Job drawing, mm, ordinate dimensions from the low corner. One solid piece. Round coordinates to 2 decimals unless told otherwise and drop trailing zeros. Write each loop counter-clockwise with the first axis right and the second up, starting at its lowest first coordinate (ties: lowest second). Pieces come first, ordered by that corner, then holes. Notation, with made-up numbers: M 4,30 L 60,30 A22 ccw 60,46 Z; hole C -29.75,-21.5 d3. An arc over 180 degrees is marked long. Answer as a JSON object with one key per item and string values. Group by question number.
1. Two-plate mould, pull along Y, no slides. Class the marked faces 1 and 2: +Y half, -Y half, draft (parallel to the pull), parting line (faces both ways), or undercut.
2. Band-saw the part on C-C, the plane z = 33. Write the cut outline in (x, y).
3. Band-saw the part on D-D, the plane y = 503. Write the cut outline in (x, z).
4. Band-saw the part on B-B, the plane x = 67. Write the cut outline in (y, z), plus the area to 3 significant figures.
5. Band-saw the part on A-A, the plane y = 200. Write the cut outline in (x, z), plus the area to 3 significant figures.
6. Drill centre lines: line 1 (Z direction, x = 118.5, y = 300); line 2 (Y direction, x = 180, z = 32); line 3 (Y direction, x = 115.5, z = 41). Where is each one in solid material? Low to high. Write a range as from..to.
7. Drop flat-ended pins along their axis: pin 1 (5 mm diameter, centred on x = 121.5, z = 40.5, fed in from +Y); pin 2 (1 mm diameter, centred on x = 165.5, z = 56, fed in from +Y); pin 3 (4 mm diameter, centred on x = 60.5, z = 46.5, fed in from +Y). Give the stop position or say it passes through.
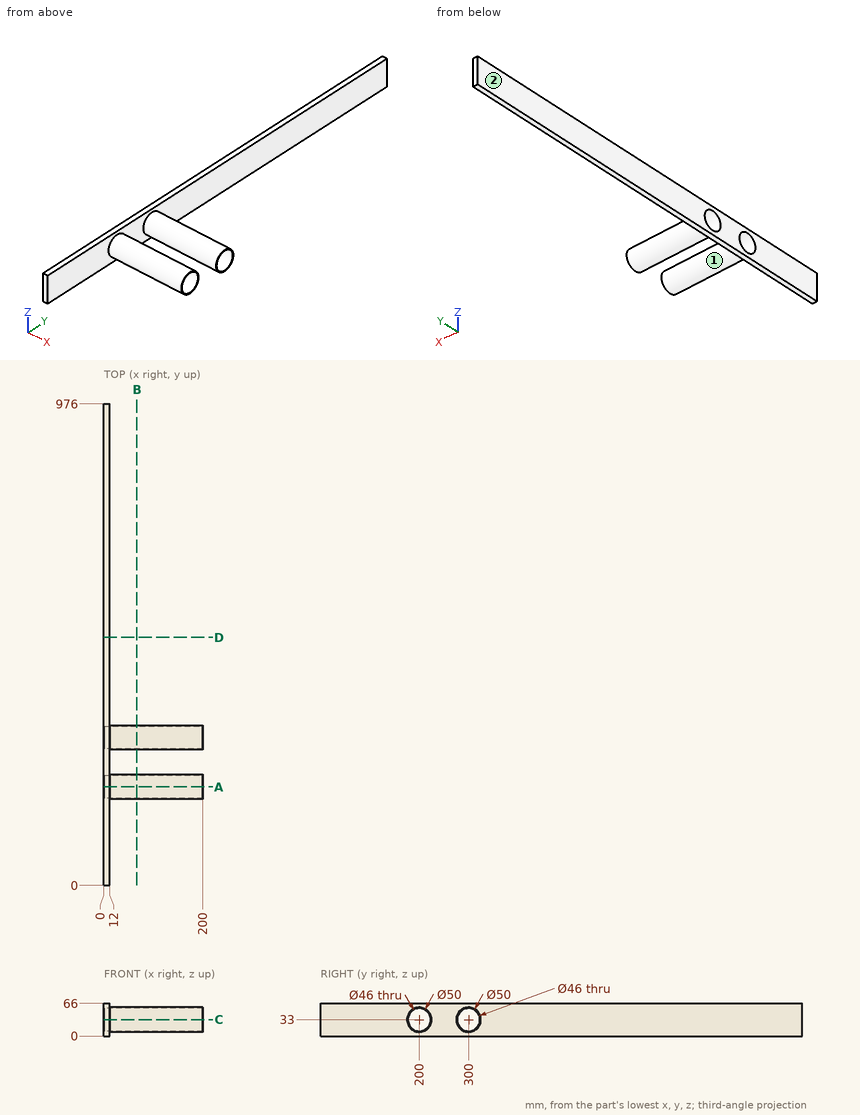
Worked answers:
{
 "1": {"face 1": "undercut", "face 2": "draft"},
 "2": {"outline": "M 0,0 L 12,0 L 12,175 L 200,175 L 200,177 L 0,177 Z; M 0,223 L 200,223 L 200,225 L 12,225 L 12,275 L 200,275 L 200,277 L 0,277 Z; M 0,323 L 200,323 L 200,325 L 12,325 L 12,976 L 0,976 Z"},
 "3": {"outline": "M 0,0 L 12,0 L 12,66 L 0,66 Z"},
 "4": {"outline": "C 200,33 d50; C 300,33 d50; hole C 200,33 d46; hole C 300,33 d46", "area": "603 mm^2"},
 "5": {"outline": "M 0,0 L 12,0 L 12,8 L 200,8 L 200,10 L 0,10 Z; M 0,56 L 200,56 L 200,58 L 12,58 L 12,66 L 0,66 Z", "area": "992 mm^2"},
 "6": {"line 1": "z = 8..10, 56..58", "line 2": "y = 175.02..177.02, 222.98..224.98, 275.02..277.02, 322.98..324.98", "line 3": "y = 176.31..178.44, 221.56..223.69, 276.31..278.44, 321.56..323.69"},
 "7": {"pin 1": "stops at y = 324.49", "pin 2": "stops at y = 310.9", "pin 3": "stops at y = 322.2"}
}
